Can you work these out from the model? Positions are in its coordinate system, mm. Face numbers are marked on the shaded views. Coordinates: 2 decimals unless noted, no trailing zeros. Loops run counter-clockwise (first coordinate to the right, second up) from the corner with the lowest first, then second, coordinate; pieces in that order, holes last.
```python
from build123d import *

# Parameters (mm, degrees)
EXTRUDE_1_DEPTH          = 10
SKETCH_2_R               = 1.5
EXTRUDE_2_DEPTH          = 5
SKETCH_3_R               = 1.5
CUT_EXTRUDE_1_DEPTH      = 16.360257159
CUT_EXTRUDE_2_DEPTH      = 11.532687216
CUT_EXTRUDE_2_DEPTH_BACK = 11.532687216
SKETCH_4_R               = 1.25


with BuildPart() as part:
    # Эскиз1 → Бобышка-Вытянуть1 (new body)
    with BuildSketch(Plane(origin=(0, 0, 0), x_dir=(1, 0, 0), z_dir=(0, 1, 0))):
        Polygon((1.25, -2.165063509), (2.5, 0), (1.25, 2.165063509), (-1.25, 2.165063509), (-2.5, 0), (-1.25, -2.165063509), align=None)
    extrude(amount=EXTRUDE_1_DEPTH)

    # Эскиз2 → Бобышка-Вытянуть2 (add)
    with BuildSketch(Plane(origin=(0, 10, 0), x_dir=(1, 0, 0), z_dir=(0, 1, 0))):
        with Locations(Location((0, 0, 0), (0, 0, 270))):
            Circle(SKETCH_2_R)
    extrude(amount=EXTRUDE_2_DEPTH)

    # Эскиз3 → Вырез-Вытянуть1 (cut, through all)
    with BuildSketch(Plane.XZ):
        with Locations(Location((0, 0, 0), (0, 0, 270))):
            Circle(SKETCH_3_R)
    extrude(amount=-CUT_EXTRUDE_1_DEPTH, mode=Mode.SUBTRACT)

    # Эскиз4 → Вырез-Вытянуть2 (cut, two sides: drawn at the far end of the back side and taken through both)
    with BuildSketch(Plane.XY.offset(-CUT_EXTRUDE_2_DEPTH_BACK)):
        with Locations((0, 5)):
            Circle(SKETCH_4_R)
    extrude(amount=CUT_EXTRUDE_2_DEPTH + CUT_EXTRUDE_2_DEPTH_BACK, mode=Mode.SUBTRACT)


solid = part.part
```
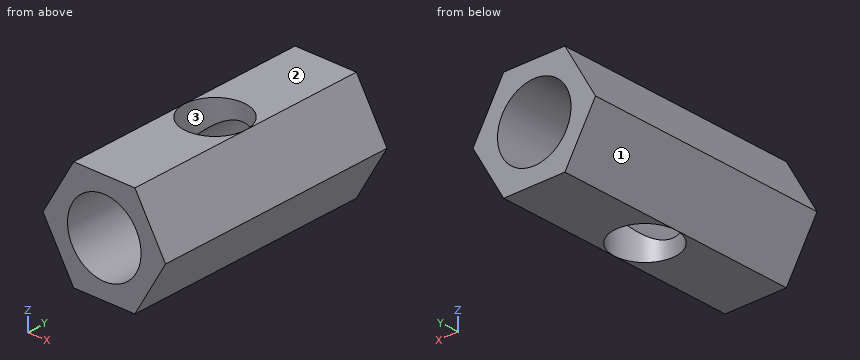
Item 1: Suppose I cut it at C-C, the plane z = 1.2. Please give me the cut outline in (x, y).
Results are:
outline: (-1.81, 0) - (-0.9, 0) - (-0.9, 4.13) arc R1.25 cw to (-0.9, 5.87) - (-0.9, 10) - (-1.81, 10) - close; (0.9, 0) - (1.81, 0) - (1.81, 10) - (0.9, 10) - (0.9, 5.87) arc R1.25 cw to (0.9, 4.13) - close
Item 2: I'm going to push flat-ended pins straight in: P1, Ø1, axis at y = 4.5, z = -1, coming from the -X side; P2, Ø1.5, axis at y = 6.5, z = -1, coming from the +X side. Where does each tip first touch, or does it pass through?
Results are:
P1: stops at x = -2.21
P2: stops at x = 2.36
Item 3: Suppose I cut it at A-A, the plane x = 0. Please give me the cut outline in (y, z), plus the area to 3 significant figures.
Results are:
outline: (0, -2.17) - (3.75, -2.17) - (3.75, -1.5) - (0, -1.5) - close; (0, 1.5) - (3.75, 1.5) - (3.75, 2.17) - (0, 2.17) - close; (6.25, -2.17) - (10, -2.17) - (10, -1.5) - (6.25, -1.5) - close; (6.25, 1.5) - (10, 1.5) - (10, 2.17) - (6.25, 2.17) - close
area: 9.98 mm2
Item 4: Suppose I cut it at B-B, the plane y = 1.25. Please give me the cut outline in (x, z), plus the area to 3 significant figures.
Results are:
outline: (-2.5, 0) - (-1.25, -2.17) - (1.25, -2.17) - (2.5, 0) - (1.25, 2.17) - (-1.25, 2.17) - close; hole circle Ø3 at (0, 0)
area: 9.17 mm2
Item 5: Suppose I cut it at D-D, the plane y = 6. Please give me the cut outline in (x, z), plus the area to 3 significant figures.
Results are:
outline: (-2.5, 0) - (-1.25, -2.17) - (-0.75, -2.17) - (-0.75, -1.3) arc R1.5 cw to (-0.75, 1.3) - (-0.75, 2.17) - (-1.25, 2.17) - close; (0.75, -2.17) - (1.25, -2.17) - (2.5, 0) - (1.25, 2.17) - (0.75, 2.17) - (0.75, 1.3) arc R1.5 cw to (0.75, -1.3) - close
area: 6.98 mm2
Item 6: We'd pull the mould along X, two halves only. Please class the marked faces 1, 2 and 3: +X half, -X half, draft (parallel to the pull), parting line (faces both ways), or undercut.
Results are:
face 1: -X half
face 2: draft
face 3: undercut
Item 7: I need wall thicknesses on line 1 along Z through (x, y) = (0, 3); line 2 along X through (y, z) = (3.25, 1.3); line 3 along X through (y, z) = (1.25, 0.95). Which ranges of each line are inside material? Lowest first, please.
Results are:
line 1: z = -2.17 to -1.5, 1.5 to 2.17
line 2: x = -1.75 to -0.75, 0.75 to 1.75
line 3: x = -1.95 to -1.16, 1.16 to 1.95
